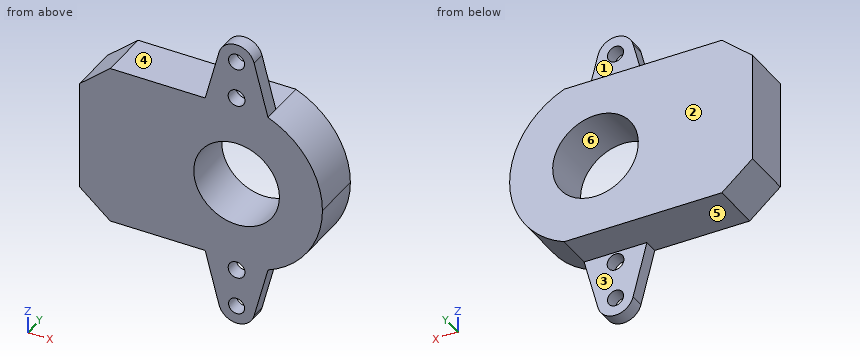
from build123d import *

# Parameters (mm, degrees)
BOSS_EXTRUDE1_DEPTH = 9
SKETCH2_R           = 1.435
SKETCH2_R_2         = 1.5
BOSS_EXTRUDE2_DEPTH = 2.54
SKETCH3_R           = 7.65
CUT_EXTRUDE1_DEPTH  = 52.496474637


with BuildPart() as part:
    # Sketch1 → Boss-Extrude1 (new body)
    with BuildSketch(Plane(origin=(0, 0, 0), x_dir=(1, 0, 0), z_dir=(0, 1, 0))):
        with BuildLine():
            Line((0, -9.7536), (0, 9.7536))
            Line((0, 9.7536), (5.464049586, 14.385))
            Line((5.464049586, 14.385), (33.652501624, 14.385))
            ThreePointArc((33.652501624, 14.385), (40.719855435, 8.682632804), (43.38, 0))
            ThreePointArc((43.38, 0), (40.719855435, -8.682632804), (33.652501624, -14.385))
            Line((33.652501624, -14.385), (5.464049586, -14.385))
            Line((5.464049586, -14.385), (0, -9.7536))
        make_face()
    extrude(amount=BOSS_EXTRUDE1_DEPTH)

    # Sketch2 → Boss-Extrude2 (add)
    # profile 1 of 2: a face of its own
    with BuildSketch(Plane.XZ):
        with BuildLine():
            Line((31.171361508, -23.834680852), (33.652501624, -14.385))
            Line((33.652501624, -14.385), (22.427498376, -14.385))
            Line((22.427498376, -14.385), (24.908638492, -23.834680852))
            ThreePointArc((24.908638492, -23.834680852), (28.04, -26.25), (31.171361508, -23.834680852))
        make_face()
        with Locations(Location((28.04, -23.0125, 0), (0, 0, 270))):
            Circle(SKETCH2_R, mode=Mode.SUBTRACT)
        with Locations(Location((28.04, -16.215, 0), (0, 0, 270))):
            Circle(SKETCH2_R_2, mode=Mode.SUBTRACT)
    # profile 2 of 2: a face of its own
    with BuildSketch(Plane.XZ):
        with BuildLine():
            Line((22.427498376, 14.385), (33.652501624, 14.385))
            Line((33.652501624, 14.385), (31.171361508, 23.834680852))
            ThreePointArc((31.171361508, 23.834680852), (28.04, 26.25), (24.908638492, 23.834680852))
            Line((24.908638492, 23.834680852), (22.427498376, 14.385))
        make_face()
        with Locations(Location((28.04, 16.215, 0), (0, 0, 270))):
            Circle(SKETCH2_R_2, mode=Mode.SUBTRACT)
        with Locations(Location((28.04, 23.0125, 0), (0, 0, 270))):
            Circle(SKETCH2_R, mode=Mode.SUBTRACT)
    extrude(amount=-BOSS_EXTRUDE2_DEPTH)

    # Sketch3 → Cut-Extrude1 (cut, through all)
    with BuildSketch(Plane(origin=(0, 9, 0), x_dir=(1, 0, 0), z_dir=(0, 1, 0))):
        with Locations(Location((28.04, 0, 0), (0, 0, 270))):
            Circle(SKETCH3_R)
    extrude(amount=-CUT_EXTRUDE1_DEPTH, mode=Mode.SUBTRACT)


solid = part.part
Can you work these out from the model? Positions are in its coordinate system, mm. Face numbers are marked on the shaded views. A direction names the side the tool comes from. Coordinates: 2 decimals unless noted, no trailing zeros. Order: outer loops, then holes, each group sorted by start corner. A loop starts at its lowest first (then second) coordinate and runs counter-clockwise, first axis right, second up. Notation, with made-up numbers: (-13.5, 34) - (15.5, 34) arc R21 ccw to (15.5, 67) - close; hole circle Ø11 at (-4.5, 73). An arc over 180 degrees is marked (long way). Answer as a JSON object with one key per item and string values. Group by question number.
Q1. On a 3-axis mill with a long thin cutter (end or side, diameter ignored), from which of +Z, -Z, +X, -X, +Y, -Y can I reach the whole of each face in a straight line? I mean the marked faces 1, 2 and 3. Say none if no direction works.
Q2. Imagine slicing it at C-C (z = 6). Please give me the cut outline in (x, y).
Q3. Imagine slicing it at D-D (z = -2.5). Please give me the cut outline in (x, y).
Q4. Will these pins go through, and if not, where does the flat tip stop? P1, Ø9, axis at x = 29.5, z = 19, coming from the +Y side; P2, Ø1, axis at y = 2, z = 11, coming from the +X side.
Q5. We'd pull the mould along Z, two halves only. Please class the marked faces 4, 5 and 6: +Z half, -Z half, draft (parallel to the pull), parting line (faces both ways), or undercut.
Q6. Imagine slicing it at B-B (x = 28.04). Give the number of separate pieces and of enclosed holes in the cut face, and give its area (3 significant figures).
Q7. I need wall thicknesses on line 1 (Z direction, x = 24, y = 6.25) (3 decimals); line 2 (X direction, y = 4.75, z = -3); line 3 (Z direction, x = 6.5, y = 3) (3 decimals). Which ranges of each line are inside material? Lowest first, please. Write a range as from..to.
Determined:
{
 "1": {"face 1": "+Z, +X, -X, +Y", "face 2": "+Z, -Z, +X, -X, +Y", "face 3": "-Z, +X, -X, +Y"},
 "2": {"outline": "(0, 0) - (23.29, 0) - (23.29, 9) - (0, 9) - close; (32.79, 0) - (42.17, 0) - (42.17, 9) - (32.79, 9) - close"},
 "3": {"outline": "(0, 0) - (20.81, 0) - (20.81, 9) - (0, 9) - close; (35.27, 0) - (43.18, 0) - (43.18, 9) - (35.27, 9) - close"},
 "4": {"P1": "stops at y = 2.54", "P2": "stops at x = 39.28"},
 "5": {"face 4": "+Z half", "face 5": "-Z half", "face 6": "undercut"},
 "6": {"separate pieces": "6", "enclosed holes": "0", "area": "152 mm2"},
 "7": {"line 1": "z = -14.385..-6.496, 6.496..14.385", "line 2": "x = 0..21, 35.08..43.09", "line 3": "z = -14.385..14.385"}
}
